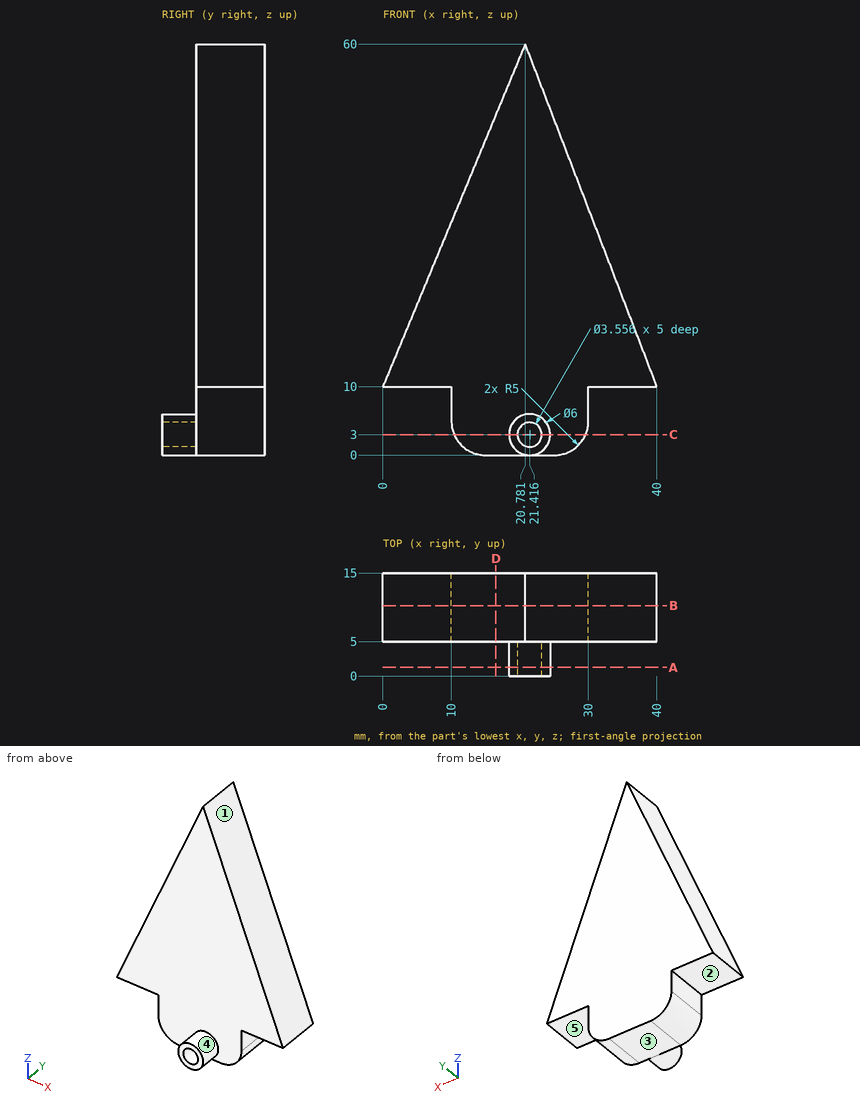
Here's the drawing with two shaded views (mm, measured from the low corner). I have some questions. A direction names the side the tool comes from. Round coordinates to 2 decimals unless told otherwise and drop trailing zeros. Loops run counter-clockwise (first coordinate to the right, second up) from the corner with the lowest first, then second, coordinate; pieces in that order, holes last. Notation, with made-up numbers: (67.5, 65.5) - (98.5, 65.5) arc R18 cw to (98.5, 79.5) - close; hole circle Ø8 at (72, 50). An arc over 180 degrees is marked (long way). Write item = value, one per line.
1) Imagine slicing it at A-A (y = 1.25). Please give me the cut outline in (x, z).
Computed:
outline = circle Ø6 at (21.42, 3); hole circle Ø3.56 at (21.42, 3)
2) I'm going to push flat-ended pins straight in: P1, Ø4, axis at y = 11.5, z = 30, coming from the +X side; P2, Ø10, axis at x = 24, z = 14.5, coming from the -Y side; P3, Ø1.5, axis at y = 7.5, z = 8.5, coming from the -X side; P4, Ø10, axis at x = 9.5, z = 48, coming from the +Y side. Where does each tip first touch, or does it pass through?
Computed:
P1 = 33.08
P2 = 5
P3 = 10
P4 = through
3) Imagine slicing it at C-C (z = 3). Please give me the cut outline in (x, y).
Computed:
outline = (10.42, 5) - (18.42, 5) - (18.42, 0) - (19.64, 0) - (19.64, 5) - (23.19, 5) - (23.19, 0) - (24.42, 0) - (24.42, 5) - (29.58, 5) - (29.58, 15) - (10.42, 15) - close
4) Imagine slicing it at B-B (y = 10.25). Please give me the cut outline in (x, z), and give its area (3 significant figures).
Computed:
outline = (0, 10) - (10, 10) - (10, 5) arc R5 ccw to (15, 0) - (25, 0) arc R5 ccw to (30, 5) - (30, 10) - (40, 10) - (20.78, 60) - close
area = 1,190 mm2
5) Imagine slicing it at D-D (x = 16.5). Please give me the cut outline in (y, z).
Computed:
outline = (5, 0) - (15, 0) - (15, 49.7) - (5, 49.7) - close
6) On a 3-axis mill with a long thin cutter (end or side, diameter ignored), from which of +Z, -Z, +X, -X, +Y, -Y can I reach the whole of each face in a straight line? I mean the marked faces 1, 2, 3, 4 and 5. Say none if no direction works.
Computed:
face_1 = +Z, +X, +Y, -Y
face_2 = -Z, -X, +Y, -Y
face_3 = -Z, +X, -X, +Y, -Y
face_4 = -Y
face_5 = -Z, +X, +Y, -Y
7) I need wall thicknesses on line 1 along X through (y, z) = (5.5, 8.5); line 2 along Z through (x, y) = (21, 4); line 3 along Y through (x, z) = (14, 25). Which ranges of each line are inside material? Lowest first, please. Write a range as from..to.
Computed:
line_1 = 10..30
line_2 = 0.03..1.27, 4.73..5.97
line_3 = 5..15
